Check sheet for the drawn part. Datum: minimum x, y, z corner. Units: mm. Round coordinates to 2 decimals unless told otherwise and drop trailing zeros. Put each result on its own line as item: value.
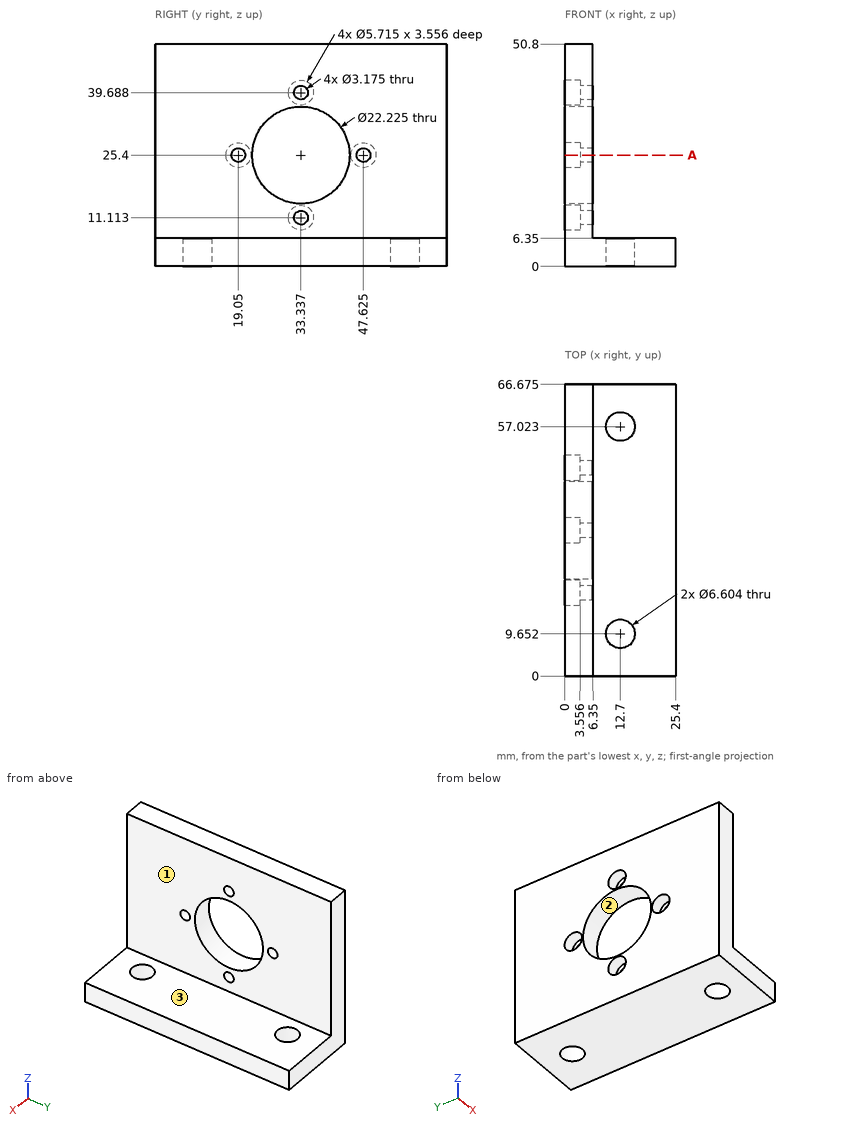
1. Cross-section at A-A (z = 25.4). Count the separate pieces of the cut face and the enclosed holes in it, then the cut area to 3 significant figures.
Computed values:
separate pieces: 4
enclosed holes: 0
area: 224 mm2
2. Release check for a two-part mould opening along Z. For the marked faces 1, 2 and 3 record: +Z half, -Z half, draft (parallel to the pull), parting line (faces both ways), or undercut.
Computed values:
face 1: draft
face 2: undercut
face 3: +Z half
3. Depth check by flat-ended pin: pin 1 Ø4.5 at (y, z) = (33.34, 11.11) entering from +X; pin 2 Ø8.5 at (x, y) = (12.7, 57.023) entering from +Z; pin 3 Ø1 at (x, z) = (2.5, 13) entering from -Y; pin 4 Ø3 at (y, z) = (46.5, 25) entering from -X. Enter the tip coordinate at first touch or a pass-through.
Computed values:
pin 1: stops at x = 6.35
pin 2: stops at z = 6.35
pin 3: stops at y = 0
pin 4: stops at x = 3.56
4. Scan lines: probe 1 along Z at (x, y) = (2.05, 19.05); probe 2 along Z at (x, y) = (5.1, 19.05); probe 3 along Z at (x, y) = (24, 59.5). Record each from-to range of solid material in increasing order.
Computed values:
probe 1: z = 0 to 22.54, 28.26 to 50.8
probe 2: z = 0 to 23.81, 26.99 to 50.8
probe 3: z = 0 to 6.35
